Build history of the part. All positions in model axes, mm. Face numbers are marked on the shaded views. A direction names the side the tool comes from. Coordinates: 2 decimals unless noted, no trailing zeros. Loops run counter-clockwise (first coordinate to the right, second up) from the corner with the lowest first, then second, coordinate; pieces in that order, holes last.
Item 1: Cut at C-C (z = 18.5). List the corners of the cut face in (x, y), and give its area (3 significant figures).
Item 2: 3-axis set-ups, long thin cutter, end or side, ignore diameter. For the marked faces 1, 2 and 3: which of +Z, -Z, +X, -X, +Y, -Y reach the whole face in a straight line?
Item 3: Cut at B-B (z = 43). List the corners of the cut face in (x, y).
Item 4: Drill centre lines: line 1 along Y through (x, z) = (-0.25, 20.5); line 2 along Z through (x, y) = (5, 12.5); line 3 along Y through (x, z) = (8, 36.15). Where is each one in solid material? Low to high.
Item 5: Flat gauge pins, fed straight in: pin 1 (1.5 mm diameter, centred on x = -10, y = -7, fed in from -Z); pin 2 (8 mm diameter, centred on x = -3, y = -6, fed in from +Z); pin 3 (3 mm diameter, centred on x = -7.5, y = -0.5, fed in from +Z). Where does each tip first touch, or does it go through?
from build123d import *

# Parameters (mm, degrees)
SKETCH1_R           = 14
BOSS_EXTRUDE1_DEPTH = 37.6
SKETCH2_R           = 5
BOSS_EXTRUDE2_DEPTH = 2.8
SKETCH3_R           = 1
BOSS_EXTRUDE3_DEPTH = 9.2
BOSS_EXTRUDE4_START = 2.6
SKETCH4_R           = 5
BOSS_EXTRUDE4_DEPTH = 2.6
BOSS_EXTRUDE5_START = 1.4
SKETCH5_R           = 1
BOSS_EXTRUDE5_DEPTH = 1.4
CHAMFER1_SIZE       = 0.3
CHAMFER2_SIZE       = 0.3
SKETCH6_R           = 1.25
CUT_EXTRUDE1_DEPTH  = 2.5
CHAMFER3_SIZE       = 0.25


with BuildPart() as part:
    # Sketch1 → Boss-Extrude1 (new body)
    with BuildSketch(Plane.XY):
        Circle(SKETCH1_R)
    extrude(amount=BOSS_EXTRUDE1_DEPTH)

    # Sketch2 → Boss-Extrude2 (add)
    with BuildSketch(Plane.XY.offset(37.6)):
        Circle(SKETCH2_R)
    extrude(amount=BOSS_EXTRUDE2_DEPTH)

    # Sketch3 → Boss-Extrude3 (add)
    with BuildSketch(Plane.XY.offset(40.4)):
        Circle(SKETCH3_R)
    extrude(amount=BOSS_EXTRUDE3_DEPTH)

    # Sketch4 → Boss-Extrude4 (add)
    with BuildSketch(Plane(origin=(0, 0, 0), x_dir=(-1, 0, 0), z_dir=(0, 0, -1)).offset(BOSS_EXTRUDE4_START)):
        with Locations(Location((0, 0, 0), (0, 0, 180))):
            Circle(SKETCH4_R)
    extrude(amount=-BOSS_EXTRUDE4_DEPTH)

    # Sketch5 → Boss-Extrude5 (add)
    with BuildSketch(Plane(origin=(0, 0, -2.6), x_dir=(-1, 0, 0), z_dir=(0, 0, -1)).offset(BOSS_EXTRUDE5_START)):
        with Locations(Location((0, 0, 0), (0, 0, 180))):
            Circle(SKETCH5_R)
    extrude(amount=-BOSS_EXTRUDE5_DEPTH)

    # Chamfer1
    chamfer1_edges = [part.edges().sort_by_distance(p)[0] for p in [
        (-5, 0, -2.6),
        (-14, 0, 37.6),
        (-5, 0, 40.4),
    ]]
    chamfer(chamfer1_edges, length=CHAMFER1_SIZE)

    # Chamfer2
    chamfer2_edges = [part.edges().sort_by_distance(p)[0] for p in [
        (-1, 0, 49.6),
        (-1, 0, -4),
    ]]
    chamfer(chamfer2_edges, length=CHAMFER2_SIZE)

    # Sketch6 → Cut-Extrude1 (cut)
    with BuildSketch(Plane.XY.offset(37.6)):
        with Locations((-8, 0)):
            Circle(SKETCH6_R)
        with Locations((8, 0)):
            Circle(SKETCH6_R)
    extrude(amount=-CUT_EXTRUDE1_DEPTH, mode=Mode.SUBTRACT)

    # Chamfer3
    chamfer3_edges = [part.edges().sort_by_distance(p)[0] for p in [
        (-9.25, 0, 37.6),
        (6.75, 0, 37.6),
    ]]
    chamfer(chamfer3_edges, length=CHAMFER3_SIZE)


solid = part.part
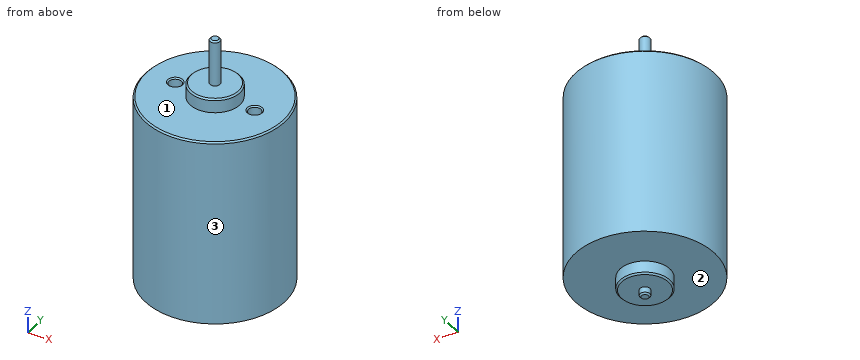
Filled sheet:
1. outline: circle Ø28 at (0, 0)
1. area: 616 mm2
2. face 1: +Z
2. face 2: -Z
2. face 3: +Z, -Z
3. outline: circle Ø2 at (0, 0)
4. line 1: y = -14 to 14
4. line 2: z = 0 to 37.6
4. line 3: y = -11.49 to -1.25, 1.25 to 11.49
5. pin 1: stops at z = 0
5. pin 2: stops at z = 40.4
5. pin 3: stops at z = 37.6
